Answer from the drawing. Dimensions are ordinates in mm from the lowest x, y and z of the part. Give positions to 0.01 mm unless a question says otherwise; leave off trailing zeros. Write each loop counter-clockwise with the first axis right and the second up, starting at its lowest first coordinate (ties: lowest second). Pieces come first, ordered by that corner, then holes. Notation, with made-up numbers: M 72.5,12.25 L 104.5,12.25 A19 ccw 104.5,41.25 Z; hole C 53.25,-14.75 d9. An arc over 180 degrees is marked long. Answer as a JSON object with one key per item and string values.
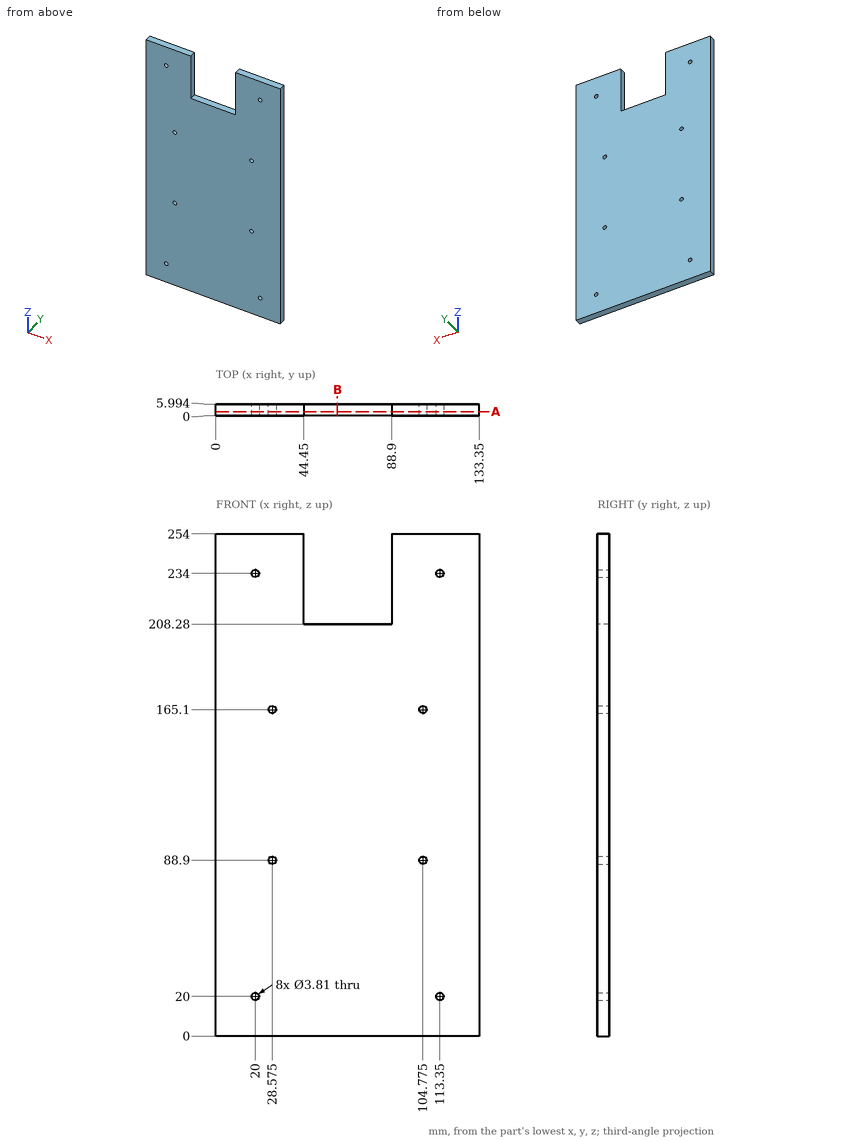
1. Flat-ended cylindrical pins translate along their axes: pin 1 (3 mm diameter, centred on x = 61.5, y = 4.5, fed in from +Z); pin 2 (2.5 mm diameter, centred on x = 28.575, z = 88.9, fed in from -Y). Find the tip coordinate at first contact, or state that the pin passes through.
Verdict:
{"pin 1": "stops at z = 208.28", "pin 2": "passes through"}
2. A cutting plane is placed at B-B, the plane x = 61.5. Give the vertices of the cut face in (y, z) (1 decimal), plus the area to 3 significant figures.
Verdict:
{"outline": "M 0,0 L 6,0 L 6,208.3 L 0,208.3 Z", "area": "1,250 mm2"}
3. A cutting plane is placed at A-A, the plane y = 2.1. Count the separate pieces of the cut face and the enclosed holes in it, plus the area to 3 significant figures.
Verdict:
{"separate pieces": "1", "enclosed holes": "8", "area": "31,700 mm2"}
4. Consider line 1 along Z through (x, y) = (113.35, 4.7) (1 decimal); line 2 along X through (y, z) = (4.4, 88.9); line 3 along Z through (x, y) = (105.5, 5.15). Determine where each line is inside the solid, lowest interval first.
Verdict:
{"line 1": "z = 0 to 18.1, 21.9 to 232.1, 235.9 to 254", "line 2": "x = 0 to 26.67, 30.48 to 102.87, 106.68 to 133.35", "line 3": "z = 0 to 87.14, 90.66 to 163.34, 166.86 to 254"}
